Autodesk Inventor part; units mm, degrees
ref_plane "YZ Plane" through (0, 0, 0) normal (1, 0, 0) x (0, 1, 0)
ref_plane "XZ Plane" through (0, 0, 0) normal (0, 1, 0) x (-1, 0, 0)
ref_plane "XY Plane" through (0, 0, 0) normal (0, 0, 1) x (1, 0, 0)
sketch "스케치1" plane through (0, 0, 0) normal (0, 0, 1) x (1, 0, 0)
  line L0 (112, -46.3919) -> (46.3919, -112)
  line L1 (46.3919, -112) -> (-46.3919, -112)
  line L2 (-46.3919, -112) -> (-112, -46.3919)
  line L3 (-112, -46.3919) -> (-112, 46.3919)
  line L4 (-112, 46.3919) -> (-46.3919, 112)
  line L5 (-46.3919, 112) -> (46.3919, 112)
  line L6 (46.3919, 112) -> (112, 46.3919)
  line L7 (112, 46.3919) -> (112, -46.3919)
  line L8 (0, 0) -> (-9.429, 0)
  line L9 (0, 0) -> (-9.429, 0)
  circle A0 centre (0, 107.302) radius 1.5
  circle A1 centre (-75.874, 75.874) radius 1.5
  circle A2 centre (-107.302, 0) radius 1.5
  circle A3 centre (-75.874, -75.874) radius 1.5
  circle A4 centre (0, -107.302) radius 1.5
  circle A5 centre (75.874, -75.874) radius 1.5
  circle A6 centre (107.302, 0) radius 1.5
  circle A7 centre (75.874, 75.874) radius 1.5
  dimension "d0" = 224
  dimension "d1" = 3
  dimension "d2" = 4.698
  dimension "d5" = 360
extrude "돌출1" add sketch "스케치1" along normal blind 5
properties part number "Cap"
CAD build for the part. Positions are in the model's coordinates, mm. Round coordinates to 2 decimals unless told otherwise and drop trailing zeros. Loops run counter-clockwise (first coordinate to the right, second up) from the corner with the lowest first, then second, coordinate; pieces in that order, holes last. Notation, with made-up numbers: (-35, 87) - (-14, 87) arc R28 ccw to (-14, 121) - close; hole circle Ø10 at (89, 48.5). An arc over 180 degrees is marked (long way). Return JSON: item names as keys, results as strings. Group by question number.
Q1. Band-saw the part on A-A on z = 0.8. Give the number of separate pieces and of enclosed holes in the cut face, plus the area to 3 significant figures.
Q2. Flat gauge pin, fed straight in: pin 1 Ø2.5 at (x, y) = (0, 107.302) entering from +Z. Where does the tip first touch, or does it go through?
Q3. Band-saw the part on C-C on x = -87. Give the cut face in (y, z).
Q4. Two-plate mould, pull along Y, no slides. Class faces 1 (the face through (-1, 112, 2)), 2 (the face through (79.655, -78.737, 2.465)), 3 (the face through (-2, 2, 0)): +Y half, -Y half, draft (parallel to the pull), parting line (faces both ways), or undercut.
Q5. Band-saw the part on B-B on y = 61. Give the cut face in (x, z).
Q6. Drill centre lines: line 1 along X through (y, z) = (-75, 4.6); line 2 along Y through (x, z) = (0, 1.5); line 3 along Y through (x, z) = (74.5, 3.2). Where is each one in solid material? Low to high. Write a range as [from, to].
Solutions:
{
 "1": {"separate pieces": "1", "enclosed holes": "8", "area": "41,500 mm^2"},
 "2": {"pin 1": "passes through"},
 "3": {"outline": "(-71.39, 0) - (71.39, 0) - (71.39, 5) - (-71.39, 5) - close"},
 "4": {"face 1": "+Y half", "face 2": "-Y half", "face 3": "draft"},
 "5": {"outline": "(-97.39, 0) - (97.39, 0) - (97.39, 5) - (-97.39, 5) - close"},
 "6": {"line 1": "x = [-83.39, -77.09], [-74.65, 74.65], [77.09, 83.39]", "line 2": "y = [-112, -108.8], [-105.8, 105.8], [108.8, 112]", "line 3": "y = [-83.89, -76.48], [-75.27, 75.27], [76.48, 83.89]"}
}
